```python
from build123d import *

# Parameters (mm, degrees)
SKETCH2_R           = 1
BOSS_EXTRUDE1_DEPTH = 3
SKETCH3_W           = 3.515258844
SKETCH3_H           = 10
BOSS_EXTRUDE2_DEPTH = 2
CHAMFER1_SIZE       = 2
FILLET1_R           = 4
FILLET2_R           = 1
CUT_EXTRUDE1_DEPTH  = 4


with BuildPart() as part:
    # Sketch2 → Boss-Extrude1 (new body)
    with BuildSketch(Plane.XY):
        with BuildLine():
            Line((47.48595993, 0.792979965), (51.48595993, 0.792979965))
            Line((51.48595993, 0.792979965), (51.48595993, 10.942979965))
            Line((51.48595993, 10.942979965), (17.68595993, 10.942979965))
            Line((17.68595993, 10.942979965), (17.68595993, 0.792979965))
            Line((17.68595993, 0.792979965), (24.68595993, 0.792979965))
            Line((24.68595993, 0.792979965), (24.68595993, 6.292979965))
            ThreePointArc((24.68595993, 6.292979965), (24.33240654, 7.146533356), (25.18595993, 6.792979965))
            Line((25.18595993, 6.792979965), (46.98595993, 6.792979965))
            ThreePointArc((46.98595993, 6.792979965), (47.839513321, 7.146533356), (47.48595993, 6.292979965))
            Line((47.48595993, 6.292979965), (47.48595993, 0.792979965))
        make_face()
        with Locations((44.48595993, 8.942979965)):
            Circle(SKETCH2_R, mode=Mode.SUBTRACT)
        with Locations((21.68595993, 8.942979965)):
            Circle(SKETCH2_R, mode=Mode.SUBTRACT)
    extrude(amount=BOSS_EXTRUDE1_DEPTH)

    # Mirror1: part across plane


with BuildPart() as part_1:
    add(part.part)
    add(part.part.mirror(Plane(origin=(0, 0.792979965, 3), x_dir=(0, 0, 1), z_dir=(0, -1, 0))))

    # Sketch3 → Boss-Extrude2 (add)
    with BuildSketch(Plane.XY.offset(3)):
        with Locations((21.943589352, 0.792979965)):
            Rectangle(SKETCH3_W, SKETCH3_H)
    extrude(amount=BOSS_EXTRUDE2_DEPTH)

    # Chamfer1
    chamfer1_edges = [part_1.edges().sort_by_distance(p)[0] for p in [
        (23.701218774, 0.792979965, 5),
    ]]
    chamfer(chamfer1_edges, length=CHAMFER1_SIZE - 0.0001)  # a hair under: the kernel refuses the full size

    # Fillet1
    fillet1_edges = [part_1.edges().sort_by_distance(p)[0] for p in [
        (51.48595993, 10.942979965, 1.5),
        (51.48595993, -9.357020035, 1.5),
    ]]
    fillet(fillet1_edges, radius=FILLET1_R)

    # Fillet2
    fillet2_edges = [part_1.edges().sort_by_distance(p)[0] for p in [
        (17.68595993, 10.942979965, 1.5),
        (17.68595993, -9.357020035, 1.5),
    ]]
    fillet(fillet2_edges, radius=FILLET2_R)

    # Sketch4 → Cut-Extrude1 (cut)
    with BuildSketch(Plane.XY.offset(3)):
        Polygon((20.18595993, -4.207020035), (17.68595993, -6.707020035), (17.68595993, 8.292979965), (20.18595993, 5.792979965), align=None)
    extrude(amount=-CUT_EXTRUDE1_DEPTH, mode=Mode.SUBTRACT)


solid = part_1.part
```
Read the model definition and answer for the solid it produces. Units are mm, in the model's axes. A direction names the side the tool comes from. Give positions to 0.01 mm unless a question says otherwise; leave off trailing zeros. Write each loop counter-clockwise with the first axis right and the second up, starting at its lowest first coordinate (ties: lowest second). Pieces come first, ordered by that corner, then holes. Notation, with made-up numbers: (-34, 87.25) -> (16, 87.25) arc R16 ccw to (16, 108.25) -> close; hole circle Ø11 at (68, 11.25). An arc over 180 degrees is marked (long way). Answer in a Markdown table with one row per item.
1) Determine the mould class of faces 5 (the flat face through (20.186, 1, 3)), 6 (the cylindrical face through (47.83, -5.57, 1.48)), 7 (the flat face through (22, 5.793, 4)) for opening direction X: released by +X, released by -X, zero draft, split by the parting line, or undercut.
Results list:
| item | result |
|---|---|
| face 5 | released by -X |
| face 6 | undercut |
| face 7 | zero draft |
2) A tool of negligible diameter and unlimited length cuts with its end or side. For faces 1 (the flat face through (22, -4.207, 4)), 2 (the flat face through (24.686, 1, 1)), 3 (the flat face through (18.953, -5.44, 1.521)), 4 (the flat face through (33, 10.943, 1)), from which of +Z, -Z, +X, -X, +Y, -Y can it reach the whole face along a straight path? Write none if from no direction.
Results list:
| item | result |
|---|---|
| face 1 | +Z, +X, -X, -Y |
| face 2 | +Z, -Z |
| face 3 | +Z, -Z, -X |
| face 4 | +Z, -Z, +X, -X, +Y |
3) Section C-C on z = 0.75 is taken. Give the vertices of the cut face in (x, y), plus the area to 3 significant figures.
Results list:
| item | result |
|---|---|
| outline | (17.69, -8.36) arc R1 ccw to (18.69, -9.36) -> (47.49, -9.36) arc R4 ccw to (51.49, -5.36) -> (51.49, 6.94) arc R4 ccw to (47.49, 10.94) -> (18.69, 10.94) arc R1 ccw to (17.69, 9.94) -> (17.69, 8.29) -> (20.19, 5.79) -> (20.19, -4.21) -> (17.69, -6.71) -> close; hole circle Ø2 at (21.69, -7.36); hole circle Ø2 at (21.69, 8.94); hole (24.69, -4.71) arc R0.5 ccw (long way) to (25.19, -5.21) -> (46.99, -5.21) arc R0.5 ccw (long way) to (47.49, -4.71) -> (47.49, 6.29) arc R0.5 ccw (long way) to (46.99, 6.79) -> (25.19, 6.79) arc R0.5 ccw (long way) to (24.69, 6.29) -> close; hole circle Ø2 at (44.49, -7.36); hole circle Ø2 at (44.49, 8.94) |
| area | 359 mm^2 |
4) Each of these flat-tipped pins is pushed along its axis until it touches: pin 1 Ø1.8 at (x, y) = (44.49, -7.36) entering from +Z; pin 2 Ø1.6 at (x, z) = (21, 4.5) entering from -Y; pin 3 Ø0.6 at (x, z) = (22, 4) entering from +Y; pin 4 Ø12 at (x, y) = (37, 5) entering from +Z. Where does it stop, or does it pass through?
Results list:
| item | result |
|---|---|
| pin 1 | through |
| pin 2 | y = -4.21 |
| pin 3 | y = 5.79 |
| pin 4 | z = 3 |
5) Section D-D on z = 3.45 is taken. Give the vertices of the cut face in (x, y), plus the area to 3 significant figures.
Results list:
| item | result |
|---|---|
| outline | (20.19, -4.21) -> (23.25, -4.21) -> (23.25, 5.79) -> (20.19, 5.79) -> close |
| area | 30.7 mm^2 |
6) Straight lines are drawn through the part: line 1 (X direction, y = 1, z = 0.85); line 2 (Y direction, x = 30.5, z = 1.35); line 3 (X direction, y = -4.5, z = 2.4). For each, find the intervals that lie inside material, in ascending order. Write a range as [from, to].
Results list:
| item | result |
|---|---|
| line 1 | [20.19, 24.69], [47.49, 51.49] |
| line 2 | [-9.36, -5.21], [6.79, 10.94] |
| line 3 | [19.89, 24.69], [47.49, 51.49] |
7) Section A-A on x = 40 is taken. Give the vertices of the cut face in (y, z), plus the area to 3 significant figures.
Results list:
| item | result |
|---|---|
| outline | (-9.36, 0) -> (-5.21, 0) -> (-5.21, 3) -> (-9.36, 3) -> close; (6.79, 0) -> (10.94, 0) -> (10.94, 3) -> (6.79, 3) -> close |
| area | 24.9 mm^2 |
